from build123d import *

# Parameters (mm, degrees)
F1_DEPTH  = 63.5
F0_W      = 25.4
F0_H      = 19.05
F2_DEPTH  = 25.4
F3_DEPTH  = 7.9375
F5_R      = 6.35
F6_R      = 15.875
F7_DEPTH  = 76.201
F8_R      = 6.35
F9_DEPTH  = 76.201
F10_R     = 3.175
F11_DEPTH = 31.75


with BuildPart() as f1:
    # F0 (on Front) → F1 (new body, symmetric)
    with BuildSketch(Plane.XZ):
        Polygon((-41.275, 9.525), (-41.275, -9.525), (41.275, -9.525), (41.275, 9.525), (22.225, 9.525), align=None)
    extrude(amount=F1_DEPTH, both=True)

    # F0 (on Front) → F2 (join, symmetric)
    with BuildSketch(Plane.XZ):
        with BuildLine():
            Line((22.225, 9.525), (41.275, 9.525))
            Line((41.275, 9.525), (41.275, 27.0002))
            ThreePointArc((41.275, 27.0002), (45.9246798487, 38.2255201513), (57.15, 42.8752))
            Line((57.15, 42.8752), (60.325, 42.8752))
            Line((60.325, 42.8752), (60.325, 61.9252))
            Line((60.325, 61.9252), (57.15, 61.9252))
            ThreePointArc((57.15, 61.9252), (32.4542956671, 51.6959043329), (22.225, 27.0002))
            Line((22.225, 27.0002), (22.225, 9.525))
        make_face()
        with Locations((73.025, 52.4002)):
            Rectangle(F0_W, F0_H)
    extrude(amount=F2_DEPTH, both=True)

    # F0 (on Front) → F3 (join, symmetric)
    with BuildSketch(Plane.XZ):
        with BuildLine():
            add(Edge.make_bspline(
                [(-41.275, 9.525), (-19.3256400526, 35.1379215717), (21.5103253722, 67.9016634822), (57.15, 61.9252)],
                knots=[0, 0, 0, 0, 111.5045361635, 111.5045361635, 111.5045361635, 111.5045361635], degree=3))
            Line((-41.275, 9.525), (22.225, 9.525))
            Line((22.225, 9.525), (22.225, 27.0002))
            ThreePointArc((22.225, 27.0002), (32.4542956671, 51.6959043329), (57.15, 61.9252))
        make_face()
    extrude(amount=F3_DEPTH, both=True)

    # F0 (on Front) → F4 (revolve)
    with BuildSketch(Plane.XZ):
        Polygon((85.725, 66.675), (85.725, 61.9252), (85.725, 42.8752), (85.725, 38.1), (111.125, 38.1), (111.125, 66.675), align=None)
    revolve(axis=Axis((85.725, 0, 52.3875), (0, 0, 1)))

    # F5
    f5_edges = [f1.edges().sort_by_distance(p)[0] for p in [
        (-41.275, -63.5, 0),
        (41.275, -63.5, 0),
        (41.275, 63.5, 0),
        (-41.275, 63.5, 0),
    ]]
    fillet(f5_edges, radius=F5_R)

    # F6 (on face) → F7 (cut, through all)
    with BuildSketch(Plane.XY.offset(66.675)):
        with Locations((85.725, 0)):
            Circle(F6_R)
    extrude(amount=-F7_DEPTH, mode=Mode.SUBTRACT)

    # F8 (on face) → F9 (cut, through all)
    with BuildSketch(Plane(origin=(0, 0, -9.525), x_dir=(1, 0, 0), z_dir=(0, 0, -1))):
        with Locations((28.575, 50.8)):
            Circle(F8_R)
        with Locations((-22.225, 50.8)):
            Circle(F8_R)
        with Locations((-22.225, -50.8)):
            Circle(F8_R)
        with Locations((28.575, -50.8)):
            Circle(F8_R)
    extrude(amount=-F9_DEPTH, mode=Mode.SUBTRACT)

    # F10 (on face) → F11 (cut, symmetric)
    with BuildSketch(Plane.XZ):
        with Locations((86.1288532615, 52.6647157967)):
            Circle(F10_R)
    extrude(amount=F11_DEPTH, both=True, mode=Mode.SUBTRACT)


solid = f1.part
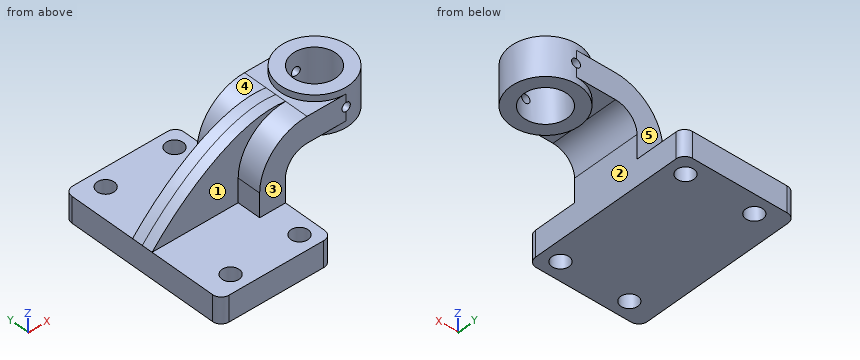
Work out the finished part from the listing and answer in its coordinate system (mm). Face numbers are marked on the shaded views. A direction names the side the tool comes from. Coordinates: 2 decimals unless noted, no trailing zeros. Write each loop counter-clockwise with the first axis right and the second up, starting at its lowest first coordinate (ties: lowest second). Pieces come first, ordered by that corner, then holes. Notation, with made-up numbers: M 27,82 L 68,82 A15 ccw 68,91 Z; hole C 22,-12.75 d9. An arc over 180 degrees is marked long. Answer as CSV lines item,"result". Start each with the question number.
Item 1: Section C-C on y = 21.5 is taken. Write down the section's boundary in (x, z) (3 decimals).
Item 2: Consider L1, parallel to X at y = -50.8, z = -4.25 (3 decimals); L2, parallel to Z at x = 64.5, y = 17; L3, parallel to Y at x = -12.5, z = 16. Determine where each line is inside the solid, lowest interval first.
Item 3: Section A-A on y = 50.8 is taken. Write down the section's boundary in (x, z) (3 decimals).
Item 4: Section D-D on y = -33.5 is taken. Write down the section's boundary in (x, z) (3 decimals).
Item 5: A tool of negligible diameter and unlimited length cuts with its end or side. For the marked faces 1, 2, 3, 4 and 5, from which of +Z, -Z, +X, -X, +Y, -Y can it reach the whole face along a straight path? Write none if from no direction.
Item 6: Flat-ended cylindrical pins translate along their axes: P1, Ø18.5, axis at y = -20.5, z = 11.5, coming from the +X side (3 decimals); P2, Ø16, axis at x = 31.5, z = 28.5, coming from the +Y side; P3, Ø5, axis at x = 86.13, z = 52.66, coming from the -Y side; P4, Ø3, axis at x = 24, y = 0, coming from the +Z side. Find the tip coordinate at first contact, or state that the pin passes through.
Item 7: Section B-B on x = 74 is taken. Write down the section's boundary in (y, z) (3 decimals), and give its area (3 significant figures).
Checks:
1,outline,"M -41.275,-9.525 L 41.275,-9.525 L 41.275,27 A15.875 cw 57.15,42.875 L 72.201,42.875 L 72.201,38.1 L 99.249,38.1 L 99.249,66.675 L 72.201,66.675 L 72.201,61.925 L 57.15,61.925 A34.925 ccw 22.225,27 L 22.225,9.525 L -41.275,9.525 Z; hole C 86.129,52.665 d6.35"
2,L1,"x = -41.275 to -28.575, -15.875 to 22.225, 34.925 to 41.275"
2,L2,"z = 42.88 to 61.93"
2,L3,"y = -7.94 to 7.94"
3,outline,"M -41.275,-9.525 L -28.575,-9.525 L -28.575,9.525 L -41.275,9.525 Z; M -15.875,-9.525 L 22.225,-9.525 L 22.225,9.525 L -15.875,9.525 Z; M 34.925,-9.525 L 41.275,-9.525 L 41.275,9.525 L 34.925,9.525 Z"
4,outline,"M -41.275,-9.525 L 41.275,-9.525 L 41.275,9.525 L -41.275,9.525 Z"
5,face 1,"+Z, -X, -Y"
5,face 2,"-Z, +X, +Y, -Y"
5,face 3,"+Z, +X, -X, -Y"
5,face 4,"+Z, -X, +Y"
5,face 5,"+Z, +X, -X, +Y"
6,P1,"stops at x = 41.275"
6,P2,"stops at y = 25.4"
6,P3,"passes through"
6,P4,"stops at z = 58.5"
7,outline,"M -25.4,42.875 L -22.532,42.875 L -22.532,38.1 L -10.702,38.1 L -10.702,66.675 L -22.532,66.675 L -22.532,61.925 L -25.4,61.925 Z; M 10.702,38.1 L 22.532,38.1 L 22.532,42.875 L 25.4,42.875 L 25.4,61.925 L 22.532,61.925 L 22.532,66.675 L 10.702,66.675 Z"
7,area,"785 mm²"
